Source: CAD feature listing. Evaluate the final solid. Frame: model axes, mm. A direction names the side the tool comes from. Give positions to 0.01 mm unless a question says otherwise; leave off trailing zeros. Order: outer loops, then holes, each group sorted by start corner. A loop starts at its lowest first (then second) coordinate and runs counter-clockwise, first axis right, second up. Notation, with made-up numbers: (31.5, 70.5) -> (85.5, 70.5) arc R24 ccw to (85.5, 88.5) -> close; hole circle Ø2 at (71.5, 15). An arc over 180 degrees is marked (long way). Answer in a Markdown table with one row per item.
```python
from build123d import *

# Parameters (mm, degrees)
SKETCH1_W            = 32.5
SKETCH1_H            = 3
SKETCH1_W_2          = 6
SKETCH1_H_2          = 7
M3_CLEARANCE_HOLE1_D = 3.4
CUT_EXTRUDE1_DEPTH   = 12.5
CIRPATTERN1_COUNT    = 14


with BuildPart() as part:
    # Sketch1 → Revolve1 (revolve)
    with BuildSketch(Plane(origin=(0, 0, 0), x_dir=(1, 0, 0), z_dir=(0, 1, 0))):
        Polygon((45, 1.5), (45, -1.5), (45, -10), (50, -10), (50, 10), (45, 10), align=None)
        with Locations((28.75, 0)):
            Rectangle(SKETCH1_W, SKETCH1_H)
        with Locations((9.5, 0)):
            Rectangle(SKETCH1_W_2, SKETCH1_H_2)
    revolve(axis=Axis((0, 0, 77.742212382), (0, 0, -1)))

    # M3 Clearance Hole1 (through all)
    with Locations(Plane.XY.offset(3.5)):
        with Locations((-4.75, 8.227241336), (4.75, 8.227241336), (9.5, 0), (4.75, -8.227241336), (-4.75, -8.227241336), (-9.5, 0)):
            Hole(M3_CLEARANCE_HOLE1_D / 2)

    # Sketch5 → Cut-Extrude1 (cut, through all)
    with BuildSketch(Plane.XY.offset(1.5)):
        with BuildLine():
            ThreePointArc((17.433407217, 1.525225498), (17.483343878, 0.763339279), (17.5, 0))
            ThreePointArc((17.5, 0), (32.3159819, 9.689882919), (29.37704918, 27.147540984))
            ThreePointArc((29.37704918, 27.147540984), (30.802914583, 10.888009592), (17.433407217, 1.525225498))
        make_face()
    cut_extrude1 = extrude(amount=-CUT_EXTRUDE1_DEPTH, mode=Mode.SUBTRACT)

    # CirPattern1: Cut-Extrude1 ×14 about axis
    cirpattern1_axis = Axis((0, 0, 0), (0, 0, 1))
    for i in range(1, CIRPATTERN1_COUNT):
        add(cut_extrude1.rotate(cirpattern1_axis, i * 360 / CIRPATTERN1_COUNT), mode=Mode.SUBTRACT)


solid = part.part
```
(1) Ray query, probe 1 along X at (y, z) = (-0.5, 6); probe 2 along X at (y, z) = (-4, 0.25); probe 3 along Z at (x, y) = (22, 38). Return the intervals inside material, ascending.
A:
| item | result |
|---|---|
| probe 1 | x = -50 to -45, 45 to 50 |
| probe 2 | x = -49.84 to -38.68, -37.65 to -28.15, -24.75 to -5.12, 5.12 to 31.91, 34.66 to 49.84 |
| probe 3 | z = -1.5 to 1.5 |
(2) Section query A-A (y = -33.5). Return the cut outline in (x, z).
A:
| item | result |
|---|---|
| outline | (-37.12, -10) -> (-30.05, -10) -> (-30.05, -1.5) -> (-20.28, -1.5) -> (-20.28, 1.5) -> (-30.05, 1.5) -> (-30.05, 10) -> (-37.12, 10) -> close; (-19.18, -1.5) -> (-11.18, -1.5) -> (-11.18, 1.5) -> (-19.18, 1.5) -> close; (-9.06, -1.5) -> (2.04, -1.5) -> (2.04, 1.5) -> (-9.06, 1.5) -> close; (5.28, -1.5) -> (30.05, -1.5) -> (30.05, -10) -> (37.12, -10) -> (37.12, 10) -> (30.05, 10) -> (30.05, 1.5) -> (5.28, 1.5) -> close |
(3) Section query B-B (z = 8). Return the cut outline in (x, y).
A:
| item | result |
|---|---|
| outline | circle Ø100 at (0, 0); hole circle Ø90 at (0, 0) |
(4) Access query for faces 1 (the flat face through (-5, 5, -3.5)), 2 (the flat face through (-5, 5, 3.5)), 3 (the cylindrical face through (-8.15, -1.03, -0.05)). Directions: +Z, -Z, +X, -X, +Y, -Y. A direction counts if a zero-diameter tool reaches every point of the face in a straight line with its end or side. Return the directions, or none.
A:
| item | result |
|---|---|
| face 1 | -Z |
| face 2 | +Z |
| face 3 | +Z, -Z |
(5) First-contact query: pin 1 Ø6 at (x, z) = (-1.5, 2.5) entering from -Y; pin 2 Ø10 at (y, z) = (-21, -3) entering from +X; pin 3 Ø3 at (x, z) = (-17.5, -4) entering from -Y. Flat tips, straight axial feed; report the tip coordinate or a pass-through.
A:
| item | result |
|---|---|
| pin 1 | stops at y = -50 |
| pin 2 | stops at x = 47.37 |
| pin 3 | stops at y = -47.37 |
(6) Section query D-D (y = 32). Return the cut outline in (x, z), plus the area to 3 significant figures.
A:
| item | result |
|---|---|
| outline | (-38.42, -10) -> (-31.64, -10) -> (-31.64, -1.5) -> (-3.2, -1.5) -> (-3.2, 1.5) -> (-31.64, 1.5) -> (-31.64, 10) -> (-38.42, 10) -> close; (-0.34, -1.5) -> (10.07, -1.5) -> (10.07, 1.5) -> (-0.34, 1.5) -> close; (12.19, -1.5) -> (20.3, -1.5) -> (20.3, 1.5) -> (12.19, 1.5) -> close; (21.59, -1.5) -> (31.64, -1.5) -> (31.64, -10) -> (38.42, -10) -> (38.42, 10) -> (31.64, 10) -> (31.64, 1.5) -> (21.59, 1.5) -> close |
| area | 442 mm^2 |
(7) Section query C-C (x = 0). Give the number of separate pieces and of enclosed holes in the cut face, plus the area to 3 significant figures.
A:
| item | result |
|---|---|
| separate pieces | 6 |
| enclosed holes | 0 |
| area | 457 mm^2 |
(8) Pull-direction query (X, two-part tool) for faces 4 (the cylindrical face through (-3.95, 32.6, 0.02)), 5 (the flat face through (-9, 9, 1.5)); classes: +X half, -X half, draft (parallel to the pull), parting line (faces both ways), or undercut.
A:
| item | result |
|---|---|
| face 4 | undercut |
| face 5 | undercut |
